Input: part model. Units: mm. Frame: model coordinates. A direction names the side the tool comes from. Coordinates: 2 decimals unless noted, no trailing zeros. Order: outer loops, then holes, each group sorted by start corner. A loop starts at its lowest first (then second) coordinate and runs counter-clockwise, first axis right, second up. Notation, with made-up numbers: (65, 48.5) -> (107, 48.5) arc R18 cw to (107, 66.5) -> close; hole circle Ø7 at (70.25, -27.5). An arc over 180 degrees is marked (long way). Write each question's results on one line, items separated by ' | '.
```python
from build123d import *

# Parameters (mm, degrees)
SKETCH_1_R          = 19.5
SKETCH_1_R_2        = 16
EXTRUDE_1_DEPTH     = 12
SKETCH_2_R          = 21
SKETCH_2_R_2        = 16
EXTRUDE_2_DEPTH     = 4
SKETCH_3_R          = 20
EXTRUDE_3_DEPTH     = 3
SKETCH_4_R          = 20
SKETCH_4_R_2        = 16
EXTRUDE_4_DEPTH     = 14
SKETCH_6_R          = 20
SKETCH_6_R_2        = 19
CUT_EXTRUDE_1_DEPTH = 1.5
CUT_EXTRUDE_START   = -3
SKETCH_7_R          = 20
CUT_EXTRUDE_2_DEPTH = 3
CHAMFER_1_SIZE      = 1
SKETCH_8_W          = 0.5
SKETCH_8_H          = 1


with BuildPart() as part:
    # 草图1 → 拉伸1 (new body)
    with BuildSketch(Plane.XY):
        Circle(SKETCH_1_R)
        Circle(SKETCH_1_R_2, mode=Mode.SUBTRACT)
    extrude(amount=EXTRUDE_1_DEPTH)

    # 草图2 → 拉伸2 (add)
    with BuildSketch(Plane.XY.offset(12)):
        Circle(SKETCH_2_R)
        Circle(SKETCH_2_R_2, mode=Mode.SUBTRACT)
    extrude(amount=EXTRUDE_2_DEPTH)

    # 草图3 → 拉伸3 (add)
    with BuildSketch(Plane.XY.offset(16)):
        Circle(SKETCH_3_R)
    extrude(amount=EXTRUDE_3_DEPTH)

    # 草图4 → 拉伸4 (add)
    with BuildSketch(Plane.XY.offset(19)):
        Circle(SKETCH_4_R)
        Circle(SKETCH_4_R_2, mode=Mode.SUBTRACT)
    extrude(amount=EXTRUDE_4_DEPTH)

    # 草图6 → 切除-拉伸1 (cut)
    with BuildSketch(Plane.XY.offset(30)):
        Circle(SKETCH_6_R)
        Circle(SKETCH_6_R_2, mode=Mode.SUBTRACT)
    extrude(amount=CUT_EXTRUDE_1_DEPTH, mode=Mode.SUBTRACT)

    # 草图7 → 切除-拉伸2 (cut)
    with BuildSketch(Plane.XY.offset(33).offset(CUT_EXTRUDE_START)):
        Circle(SKETCH_7_R)
    extrude(amount=CUT_EXTRUDE_2_DEPTH, mode=Mode.SUBTRACT)

    # 倒角1
    chamfer_1_edges = [part.edges().sort_by_distance(p)[0] for p in [
        (-20, 0, 30),
    ]]
    chamfer(chamfer_1_edges, length=CHAMFER_1_SIZE)

    # 草图8 → 切除-旋转1 (revolve, cut)
    with BuildSketch(Plane(origin=(0, 0, 0), x_dir=(1, 0, 0), z_dir=(0, 1, 0))):
        with Locations((-19.75, -16.5)):
            Rectangle(SKETCH_8_W, SKETCH_8_H)
    revolve(axis=Axis((0, 0, 0), (0, 0, 1)), mode=Mode.SUBTRACT)


solid = part.part
```
(1) Line query: line 1 along Y through (x, z) = (0, 6.75); line 2 along Z through (x, y) = (-13, -0.5); line 3 along X through (y, z) = (14, 26). Output: solid intervals per line, ascending. Write a range as from..to.
Return value:
line 1: -19.5..-16, 16..19.5 | line 2: 16..19 | line 3: -14.28..-7.75, 7.75..14.28
(2) Reachability of faces 4 (the face through (3, 16, 0)), 5 (the face through (0, 0, 19)), 6 (the face through (0, 0, 16)), 7 (the face through (2.539, -19.334, 16.493)), 8 (the face through (-10, -13, 30)) from +Z, -Z, +X, -X, +Y, -Y: full face, straight path, thin tool, end or side. Return the list, or none.
Return value:
face 4: -Z, +X, -X, +Y, -Y | face 5: +Z | face 6: -Z | face 7: none | face 8: +Z, +X, -X, +Y, -Y
(3) Cut plane A-A, the plane y = 0. Return loops of the section in (x, z), plus the area to 3 significant figures.
Return value:
outline: (-21, 12) -> (-19.5, 12) -> (-19.5, 0) -> (-16, 0) -> (-16, 16) -> (16, 16) -> (16, 0) -> (19.5, 0) -> (19.5, 12) -> (21, 12) -> (21, 16) -> (19.5, 16) -> (19.5, 17) -> (20, 17) -> (20, 29) -> (19, 30) -> (16, 30) -> (16, 19) -> (-16, 19) -> (-16, 30) -> (-19, 30) -> (-20, 29) -> (-20, 17) -> (-19.5, 17) -> (-19.5, 16) -> (-21, 16) -> close | area: 330 mm2
(4) Mould query, pull axis Z, two halves, no side actions, for faces 1 (the face through (20.03, 6.31, 13.97)), 2 (the face through (-6, 19, 16)), 3 (the face through (6, -19, 12)). Classes: +Z half, -Z half, draft (parallel to the pull), parting line (faces both ways), or undercut.
Return value:
face 1: draft | face 2: undercut | face 3: -Z half
(5) Cut plane C-C, the plane z = 25. Return loops of the section in (x, y).
Return value:
outline: circle Ø40 at (0, 0); hole circle Ø32 at (0, 0)
(6) Pin query (flat end, axial travel): P1, Ø1.5, axis at x = -15, z = 24.5, coming from the +Y side; P2, Ø1, axis at x = 10, z = 21.5, coming from the -Y side; P3, Ø12, axis at x = 1.5, y = -1, coming from the -Z side. Return the tip coordinate at first contact, or that it passes through.
Return value:
P1: y = 14.03 | P2: y = -17.6 | P3: z = 16
